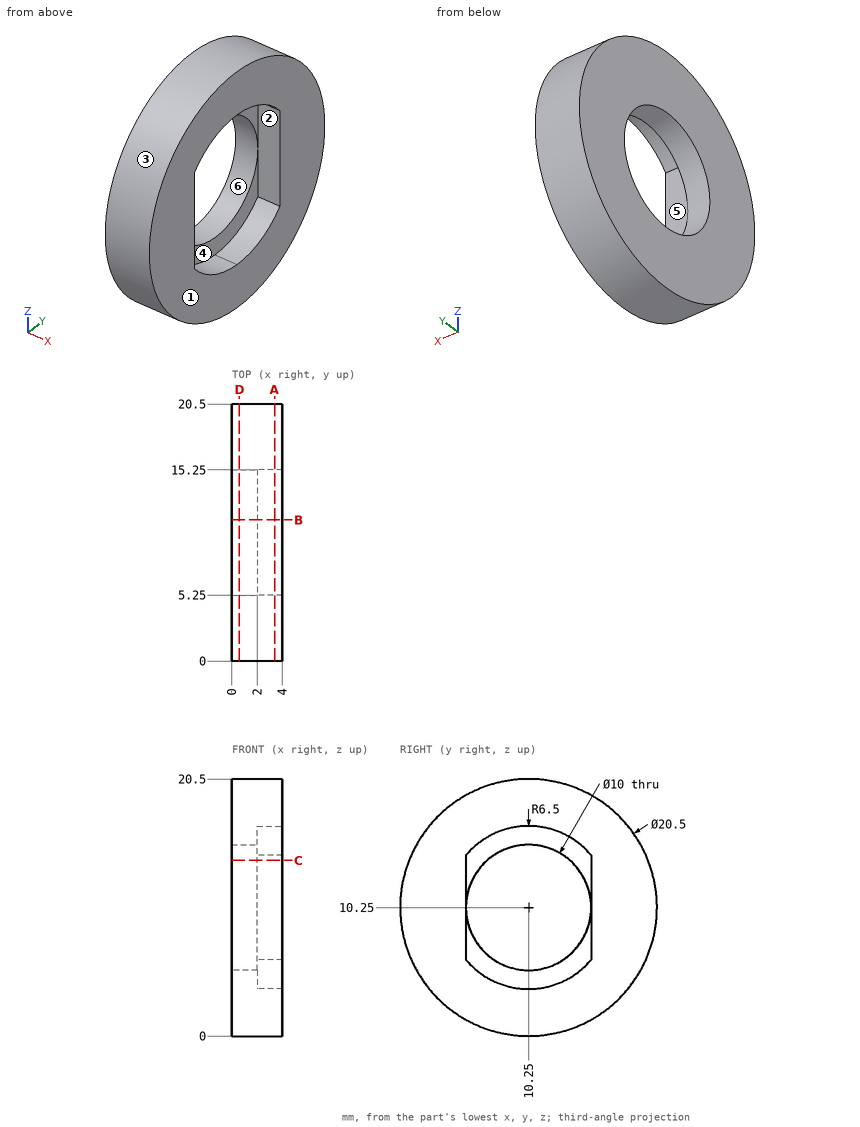
Source: three-view drawing plus pictorial views. Frame: mm from the lowest corner of the part. A direction names the side the tool comes from. Round coordinates to 2 decimals unless told otherwise and drop trailing zeros. Order: outer loops, then holes, each group sorted by start corner. A loop starts at its lowest first (then second) coordinate and runs counter-clockwise, first axis right, second up. Notation, with made-up numbers: M 74.25,0 L 101.25,0 A15 cw 101.25,7 Z; hole C 64.25,64.25 d11. An arc over 180 degrees is marked long. One line per item, written item: value.
(1) Pull-direction query (Y, two-part tool) for the marked faces 1, 2, 3 and 4; classes: pulls with the +Y half, pulls with the -Y half, needs draft (parallel to the pull), parting line crosses it, or undercut.
Result sheet:
face 1: needs draft
face 2: undercut
face 3: parting line crosses it
face 4: undercut
(2) Cut plane B-B (y = 11.25). Return the cut outline in (x, z), and give its area (3 significant figures).
Result sheet:
outline: M 0,0.05 L 4,0.05 L 4,3.83 L 2,3.83 L 2,5.35 L 0,5.35 Z; M 0,15.15 L 2,15.15 L 2,16.67 L 4,16.67 L 4,20.45 L 0,20.45 Z
area: 36.3 mm2
(3) Line query: probe 1 along Y at (x, z) = (0.55, 10.25); probe 2 along Y at (x, z) = (2.15, 8); probe 3 along Z at (x, y) = (1.55, 13.5). Output: solid intervals per line, ascending. Write a range as [from, to].
Result sheet:
probe 1: [0, 5.25], [15.25, 20.5]
probe 2: [0.25, 5.25], [15.25, 20.25]
probe 3: [0.53, 6.45], [14.05, 19.97]
(4) Cut plane A-A (x = 3.4). Return the cut outline in (y, z).
Result sheet:
outline: C 10.25,10.25 d20.5; hole M 5.25,6.1 A6.5 ccw 15.25,6.1 L 15.25,14.4 A6.5 ccw 5.25,14.4 Z
(5) Pin query (flat end, axial travel): P1, Ø0.6, axis at x = 3, z = 9, coming from the +Y side; P2, Ø3.5, axis at y = 12.5, z = 13, coming from the +X side; P3, Ø1.5, axis at x = 0.5, z = 8, coming from the +Y side. Return the tip coordinate at first contact, or that it passes through.
Result sheet:
P1: y = 20.46
P2: x = 2
P3: y = 20.39
(6) Cut plane C-C (z = 14). Return the cut outline in (x, y).
Result sheet:
outline: M 0,0.71 L 4,0.71 L 4,5.25 L 2,5.25 L 2,6.94 L 0,6.94 Z; M 0,13.56 L 2,13.56 L 2,15.25 L 4,15.25 L 4,19.79 L 0,19.79 Z
(7) Cut plane D-D (x = 0.6). Return the cut outline in (y, z).
Result sheet:
outline: C 10.25,10.25 d20.5; hole C 10.25,10.25 d10
(8) Reachability of the marked faces 5 and 6 from +Z, -Z, +X, -X, +Y, -Y: full face, straight path, thin tool, end or side. Return the list, or none.
Result sheet:
face 5: +X
face 6: +X, -X
